```python
from build123d import *

# Parameters (mm, degrees)
BASE_PLATE_AND_PORTS_2_R   = 0.35
BASE_PLATE_AND_PORTS_2_R_2 = 1.05
BASE_PLATE_AND_PORTS_DEPTH = 1.5
RESERVOIRS_W               = 0.5
RESERVOIRS_H               = 12
BOSS_EXTRUDE1_DEPTH        = 15


with BuildPart() as part:
    # Base-plate and ports 2 → Base plate and ports (new, symmetric)
    with BuildSketch(Plane(origin=(0, 0, 0), x_dir=(1, 0, 0), z_dir=(0, 1, 0))):
        with BuildLine():
            Line((-16, -7), (-16, 7))
            ThreePointArc((-16, 7), (-15.560660172, 8.060660172), (-14.5, 8.5))
            Line((-14.5, 8.5), (-3.175, 8.5))
            ThreePointArc((-3.175, 8.5), (-2.379504871, 8.829504871), (-2.05, 9.625))
            ThreePointArc((-2.05, 9.625), (0, 11.675), (2.05, 9.625))
            ThreePointArc((2.05, 9.625), (2.379504871, 8.829504871), (3.175, 8.5))
            Line((3.175, 8.5), (14.5, 8.5))
            ThreePointArc((14.5, 8.5), (15.560660172, 8.060660172), (16, 7))
            Line((16, 7), (16, -7))
            ThreePointArc((16, -7), (15.560660172, -8.060660172), (14.5, -8.5))
            Line((14.5, -8.5), (12.175, -8.5))
            ThreePointArc((12.175, -8.5), (11.379504871, -8.829504871), (11.05, -9.625))
            ThreePointArc((11.05, -9.625), (9, -11.675), (6.95, -9.625))
            ThreePointArc((6.95, -9.625), (6.620495129, -8.829504871), (5.825, -8.5))
            Line((5.825, -8.5), (-5.825, -8.5))
            ThreePointArc((-5.825, -8.5), (-6.620495129, -8.829504871), (-6.95, -9.625))
            ThreePointArc((-6.95, -9.625), (-9, -11.675), (-11.05, -9.625))
            ThreePointArc((-11.05, -9.625), (-11.379504871, -8.829504871), (-12.175, -8.5))
            Line((-12.175, -8.5), (-14.5, -8.5))
            ThreePointArc((-14.5, -8.5), (-15.560660172, -8.060660172), (-16, -7))
        make_face()
        with Locations(Location((-10.5, 3, 0), (0, 0, 270))):
            Circle(BASE_PLATE_AND_PORTS_2_R, mode=Mode.SUBTRACT)
        with Locations(Location((10.5, 3, 0), (0, 0, 270))):
            Circle(BASE_PLATE_AND_PORTS_2_R, mode=Mode.SUBTRACT)
        with Locations(Location((10.5, -3, 0), (0, 0, 270))):
            Circle(BASE_PLATE_AND_PORTS_2_R, mode=Mode.SUBTRACT)
        with Locations(Location((-10.5, -3, 0), (0, 0, 270))):
            Circle(BASE_PLATE_AND_PORTS_2_R, mode=Mode.SUBTRACT)
        with Locations(Location((0, 9.625, 0), (0, 0, 270))):
            Circle(BASE_PLATE_AND_PORTS_2_R_2, mode=Mode.SUBTRACT)
        with Locations(Location((-9, -9.625, 0), (0, 0, 270))):
            Circle(BASE_PLATE_AND_PORTS_2_R_2, mode=Mode.SUBTRACT)
        with Locations(Location((9, -9.625, 0), (0, 0, 270))):
            Circle(BASE_PLATE_AND_PORTS_2_R_2, mode=Mode.SUBTRACT)
    extrude(amount=BASE_PLATE_AND_PORTS_DEPTH, both=True)

    # Reservoirs → Boss-Extrude1 (add)
    # profile 1 of 2: a face of its own
    with BuildSketch(Plane(origin=(0, 1.5, 0), x_dir=(1, 0, 0), z_dir=(0, 1, 0))):
        with BuildLine():
            Line((-13.5, 6.5), (13.5, 6.5))
            ThreePointArc((13.5, 6.5), (13.853553391, 6.353553391), (14, 6))
            Line((14, 6), (14, -6))
            ThreePointArc((14, -6), (13.853553391, -6.353553391), (13.5, -6.5))
            Line((13.5, -6.5), (-13.5, -6.5))
            ThreePointArc((-13.5, -6.5), (-13.853553391, -6.353553391), (-14, -6))
            Line((-14, -6), (-14, 6))
            ThreePointArc((-14, 6), (-13.853553391, 6.353553391), (-13.5, 6.5))
        make_face()
        Polygon((4.333333333, -6), (4.833333333, -6), (13.5, -6), (13.5, 6), (4.833333333, 6), (4.333333333, 6), (-4.333333333, 6), (-4.833333333, 6), (-13.5, 6), (-13.5, -6), (-4.833333333, -6), (-4.333333333, -6), align=None, mode=Mode.SUBTRACT)
    # profile 2 of 2: a face of its own
    with BuildSketch(Plane(origin=(0, 1.5, 0), x_dir=(1, 0, 0), z_dir=(0, 1, 0))):
        Rectangle(RESERVOIRS_W, RESERVOIRS_H)
    extrude(amount=BOSS_EXTRUDE1_DEPTH)


solid = part.part
```
The model under review builds one solid part; all positions refer to its coordinate system, in mm. A direction names the side the tool comes from. Round coordinates to 2 decimals unless told otherwise and drop trailing zeros. Loops run counter-clockwise (first coordinate to the right, second up) from the corner with the lowest first, then second, coordinate; pieces in that order, holes last.
Item 1: For line 1 (X direction, y = -0.9, z = 3); line 2 (X direction, y = 7.25, z = -1.5); line 3 (Z direction, x = -6, y = 11), list the stretches that pass through material, from the lowest coordinate up.
Determined:
line 1: x = -16 to -10.85, -10.15 to 10.15, 10.85 to 16
line 2: x = -14 to -13.5, -0.25 to 0.25, 13.5 to 14
line 3: z = -6.5 to -6, 6 to 6.5
Item 2: Take a section at C-C (y = 3). Write out the cut boundary in (x, z), then the cut area to 3 significant figures.
Determined:
outline: (-14, -6) arc R0.5 ccw to (-13.5, -6.5) - (13.5, -6.5) arc R0.5 ccw to (14, -6) - (14, 6) arc R0.5 ccw to (13.5, 6.5) - (-13.5, 6.5) arc R0.5 ccw to (-14, 6) - close; hole (-13.5, -6) - (-0.25, -6) - (-0.25, 6) - (-13.5, 6) - close; hole (0.25, -6) - (13.5, -6) - (13.5, 6) - (0.25, 6) - close
area: 45.8 mm2
Item 3: For faces 1 (the face through (14, 9, 0)), 2 (the face through (0, 9, 6.5)), 3 (the face through (0, 0, 8.5)), 4 (the face through (7, 9, -6)), 5 (the face through (-14, 9, 0)), list the 3-axis set-ups (+Z, -Z, +X, -X, +Y, -Y) from which the entire face can be reached by the end or side of a thin tool; tool diameter is ignored.
Determined:
face 1: +Z, -Z, +X, +Y
face 2: +Z, +X, -X, +Y
face 3: +Z, +Y, -Y
face 4: +Y
face 5: +Z, -Z, -X, +Y
Item 4: Take a section at B-B (x = -9). Write out the cut boundary in (y, z) (3 decimals), then the cut area to 3 significant figures.
Determined:
outline: (-1.5, -8.5) - (1.5, -8.5) - (1.5, -6.5) - (16.5, -6.5) - (16.5, -6) - (1.5, -6) - (1.5, 6) - (16.5, 6) - (16.5, 6.5) - (1.5, 6.5) - (1.5, 8.575) - (-1.5, 8.575) - close; (-1.5, 10.675) - (1.5, 10.675) - (1.5, 11.675) - (-1.5, 11.675) - close
area: 69.2 mm2
Item 5: Take a section at D-D (y = 0.25). Write out the cut boundary in (x, z) (3 decimals).
Determined:
outline: (-16, -7) arc R1.5 ccw to (-14.5, -8.5) - (-3.175, -8.5) arc R1.125 cw to (-2.05, -9.625) arc R2.05 ccw to (2.05, -9.625) arc R1.125 cw to (3.175, -8.5) - (14.5, -8.5) arc R1.5 ccw to (16, -7) - (16, 7) arc R1.5 ccw to (14.5, 8.5) - (12.175, 8.5) arc R1.125 cw to (11.05, 9.625) arc R2.05 ccw to (6.95, 9.625) arc R1.125 cw to (5.825, 8.5) - (-5.825, 8.5) arc R1.125 cw to (-6.95, 9.625) arc R2.05 ccw to (-11.05, 9.625) arc R1.125 cw to (-12.175, 8.5) - (-14.5, 8.5) arc R1.5 ccw to (-16, 7) - close; hole circle Ø0.7 at (-10.5, -3); hole circle Ø0.7 at (-10.5, 3); hole circle Ø2.1 at (-9, 9.625); hole circle Ø2.1 at (0, -9.625); hole circle Ø2.1 at (9, 9.625); hole circle Ø0.7 at (10.5, -3); hole circle Ø0.7 at (10.5, 3)
Item 6: Clearance check with flat-ended pins moving along their axes: pin 1 Ø1.7 at (x, z) = (9, 9.625) entering from -Y; pin 2 Ø4 at (x, y) = (8, 6.5) entering from -Z; pin 3 Ø2.5 at (x, z) = (-9, 9.625) entering from +Y; pin 4 Ø9.5 at (y, z) = (10.5, -1.5) entering from +X. State where each tip first meets the part, or that it passes through.
Determined:
pin 1: passes through
pin 2: stops at z = -6.5
pin 3: stops at y = 1.5
pin 4: stops at x = 14
Item 7: Take a section at A-A (z = 3). Write out the cut boundary in (x, y).
Determined:
outline: (-16, -1.5) - (-10.85, -1.5) - (-10.85, 1.5) - (-13.5, 1.5) - (-13.5, 16.5) - (-14, 16.5) - (-14, 1.5) - (-16, 1.5) - close; (-10.15, -1.5) - (10.15, -1.5) - (10.15, 1.5) - (0.25, 1.5) - (0.25, 16.5) - (-0.25, 16.5) - (-0.25, 1.5) - (-10.15, 1.5) - close; (10.85, -1.5) - (16, -1.5) - (16, 1.5) - (14, 1.5) - (14, 16.5) - (13.5, 16.5) - (13.5, 1.5) - (10.85, 1.5) - close
Item 8: Mouldability with a two-part tool opening along X and no side actions: class faces 6 (the face through (15.57, 0.02, 8.05)), 7 (the face through (0, 9, -6.5)), 8 (the face through (13.5, 9, 0)), 9 (the face through (-2.39, 0.02, -8.82)) as released by +X, released by -X, zero draft, split by the parting line, or undercut.
Determined:
face 6: released by +X
face 7: zero draft
face 8: undercut
face 9: released by -X
